```python
from build123d import *

# Parameters (mm, degrees)
F0_R     = 8
F1_DEPTH = 25
F2_W     = 16
F2_H     = 16
F3_DEPTH = 10
F4_W     = 1
F4_H     = 8
F5_DEPTH = 10
F6_W     = 2.5
F6_H     = 8
F7_DEPTH = 5


with BuildPart() as f1:
    # F0 (on Front) → F1 (new body)
    with BuildSketch(Plane.XZ):
        Circle(F0_R)
    extrude(amount=F1_DEPTH)

    # F2 (on face) → F3 (join)
    with BuildSketch(Plane.XZ):
        Rectangle(F2_W, F2_H)
    extrude(amount=-F3_DEPTH)

    # F4 (on face) → F5 (join)
    with BuildSketch(Plane(origin=(0, 10, 0), x_dir=(-1, 0, 0), z_dir=(0, 1, 0))):
        with Locations((2.5, 0)):
            Rectangle(F4_W, F4_H)
        with Locations((-2.5, 0)):
            Rectangle(F4_W, F4_H)
    extrude(amount=F5_DEPTH)

    # F6 (on face) → F7 (join)
    with BuildSketch(Plane(origin=(0, 20, 0), x_dir=(-1, 0, 0), z_dir=(0, 1, 0))):
        with Locations((3.25, 0)):
            Rectangle(F6_W, F6_H)
        with Locations((-3.25, 0)):
            Rectangle(F6_W, F6_H)
    extrude(amount=-F7_DEPTH)


solid = f1.part
```
Geometry check sheet. Reference: the model listing, model coordinates, mm. A direction names the side the tool comes from. Give positions to 0.01 mm unless a question says otherwise; leave off trailing zeros. Write each loop counter-clockwise with the first axis right and the second up, starting at its lowest first coordinate (ties: lowest second). Pieces come first, ordered by that corner, then holes. Notation, with made-up numbers: (-9.5, 18) -> (37.5, 18) arc R15 ccw to (37.5, 40) -> close; hole circle Ø4 at (-21, 36.25). An arc over 180 degrees is marked (long way). One line per question, with ' | ' between items.
Item 1: Sectioned sample at C-C, the plane x = -1.5. Record the boundary of the cut face in (y, z), plus the area to 3 significant figures.
Determined:
outline: (-25, -7.86) -> (0, -7.86) -> (0, -8) -> (10, -8) -> (10, 8) -> (0, 8) -> (0, 7.86) -> (-25, 7.86) -> close | area: 553 mm^2
Item 2: Sectioned sample at A-A, the plane y = 12.5. Record the boundary of the cut face in (x, z), plus the area to 3 significant figures.
Determined:
outline: (-3, -4) -> (-2, -4) -> (-2, 4) -> (-3, 4) -> close; (2, -4) -> (3, -4) -> (3, 4) -> (2, 4) -> close | area: 16.0 mm^2
Item 3: Draft check along X on faces 1 (the flat face through (3, 20, 0)), 2 (the flat face through (-2, 15, 0)), 3 (the flat face through (-8, 5, 0)). Enter one of: released by +X, released by -X, zero draft, split by the parting line, or undercut.
Determined:
face 1: zero draft | face 2: undercut | face 3: released by -X
Item 4: Sectioned sample at D-D, the plane y = -12. Record the boundary of the cut face in (x, z), plus the area to 3 significant figures.
Determined:
outline: circle Ø16 at (0, 0) | area: 201 mm^2
Item 5: Sectioned sample at B-B, the plane z = -3.5. Record the boundary of the cut face in (x, y).
Determined:
outline: (-8, 0) -> (-7.19, 0) -> (-7.19, -25) -> (7.19, -25) -> (7.19, 0) -> (8, 0) -> (8, 10) -> (3, 10) -> (3, 15) -> (4.5, 15) -> (4.5, 20) -> (2, 20) -> (2, 10) -> (-2, 10) -> (-2, 20) -> (-4.5, 20) -> (-4.5, 15) -> (-3, 15) -> (-3, 10) -> (-8, 10) -> close
Item 6: Scan lines: line 1 along Y through (x, z) = (-3.25, 0.5); line 2 along Y through (x, z) = (7, -1); line 3 along Z through (x, y) = (5, -0.5) (3 decimals). Record each from-to range of solid material in increasing order.
Determined:
line 1: -25 to 10, 15 to 20 | line 2: -25 to 10 | line 3: -6.245 to 6.245
Item 7: Depth check by flat-ended pin: pin 1 (9 mm diameter, centred on y = 16, z = 0, fed in from -X); pin 2 (3 mm diameter, centred on x = -3, y = 14, fed in from +Z); pin 3 (6 mm diameter, centred on x = -4.5, y = -14, fed in from +Z). Enter the tip coordinate at first touch or a pass-through.
Determined:
pin 1: x = -4.5 | pin 2: z = 4 | pin 3: z = 7.86
Item 8: Access from +Z, -Z, +X, -X, +Y, -Y to the whole of each face (thin tool, end or side, straight path). Record for faces 4 (the flat face through (-6, 0, -6)), 5 (the flat face through (-4, 15, 0)), 6 (the flat face through (-4.5, 18, 0)), 7 (the flat face through (2, 15, 0)), 8 (the flat face through (6, 0, 6)).
Determined:
face 4: -Z, -X, -Y | face 5: +Z, -Z, -X | face 6: +Z, -Z, -X, +Y | face 7: +Z, -Z, +Y | face 8: +Z, +X, -Y
